from build123d import *

# Parameters (mm, degrees)
F0_W     = 35.6490109116
F0_H     = 18.6256058514
F1_DEPTH = 127
F2_R     = 6.8542963407
F3_DEPTH = 25.4
F4_R     = 5.08
F5_SIZE  = 5.07999


# Not quite as in the source:
# - a fillet or chamfer is up to 0.001 mm smaller than in the source, because OpenCascade refuses the exact size


with BuildPart() as f1:
    # F0 (on Right) → F1 (new body)
    with BuildSketch(Plane.YZ):
        with Locations((-41.2567211315, -34.4473589212)):
            Rectangle(F0_W, F0_H)
    extrude(amount=F1_DEPTH)

    # F2 (on face) → F3 (cut)
    with BuildSketch(Plane.XY.offset(-25.1345559955)):
        with Locations((75.5256735351, -37.2293450889)):
            Circle(F2_R)
    extrude(amount=-F3_DEPTH, mode=Mode.SUBTRACT)

    # F4
    f4_edges = [f1.edges().sort_by_distance(p)[0] for p in [
        (0, -41.256721, -25.134556),
    ]]
    fillet(f4_edges, radius=F4_R)

    # F5 (size 5.08 in the source; OpenCascade refuses exactly that, so slightly less here)
    f5_edges = [f1.edges().sort_by_distance(p)[0] for p in [
        (66.04, -59.081227, -25.134556),
    ]]
    chamfer(f5_edges, length=F5_SIZE)


solid = f1.part
Part model, mm, in its own coordinate system. Give positions to 0.01 mm unless a question says otherwise; leave off trailing zeros. Loops run counter-clockwise (first coordinate to the right, second up) from the corner with the lowest first, then second, coordinate; pieces in that order, holes last.
(1) Band-saw the part on B-B (y = -36). Write the cut outline in (x, z).
Return value:
outline: (0, -43.76) - (68.78, -43.76) - (68.78, -25.13) - (5.08, -25.13) arc R5.08 ccw to (0, -30.21) - close; (82.27, -43.76) - (127, -43.76) - (127, -25.13) - (82.27, -25.13) - close
(2) Band-saw the part on A-A (x = 76). Write the cut outline in (y, z), and give its area (3 significant figures).
Return value:
outline: (-59.08, -43.76) - (-44.07, -43.76) - (-44.07, -25.13) - (-54, -25.13) - (-59.08, -30.21) - close; (-30.39, -43.76) - (-23.43, -43.76) - (-23.43, -25.13) - (-30.39, -25.13) - close
area: 396 mm2
(3) Pull direction X, two halves, no side cores. Call faces 1 (the flat face through (0, -39, -37)), 2 (the cylindrical face through (78.69, -43.31, -34.32)), 3 (the flat face through (63, -42, -43.76)): pulls with the +X half, pulls with the -X half, needs draft (parallel to the pull), parting line crosses it, or undercut.
Return value:
face 1: pulls with the -X half
face 2: undercut
face 3: needs draft
(4) Drill centre lines: line 1 along Y through (x, z) = (76, -38.5); line 2 along X through (y, z) = (-37, -32.5); line 3 along Y through (x, z) = (81, -32.5). Where is each one in solid material? Low to high.
Return value:
line 1: y = -59.08 to -44.07, -30.39 to -23.43
line 2: x = 0 to 68.68, 82.38 to 127
line 3: y = -59.08 to -41.35, -33.1 to -23.43
(5) Band-saw the part on C-C (z = -39). Write the cut outline in (x, y), and give its area (3 significant figures).
Return value:
outline: (0, -54) - (5.08, -59.08) - (127, -59.08) - (127, -23.43) - (0, -23.43) - close; hole circle Ø13.71 at (75.53, -37.23)
area: 4,370 mm2
(6) Band-saw the part on D-D (x = 17.5). Write the cut outline in (y, z), and give its area (3 significant figures).
Return value:
outline: (-59.08, -43.76) - (-23.43, -43.76) - (-23.43, -25.13) - (-54, -25.13) - (-59.08, -30.21) - close
area: 651 mm2
